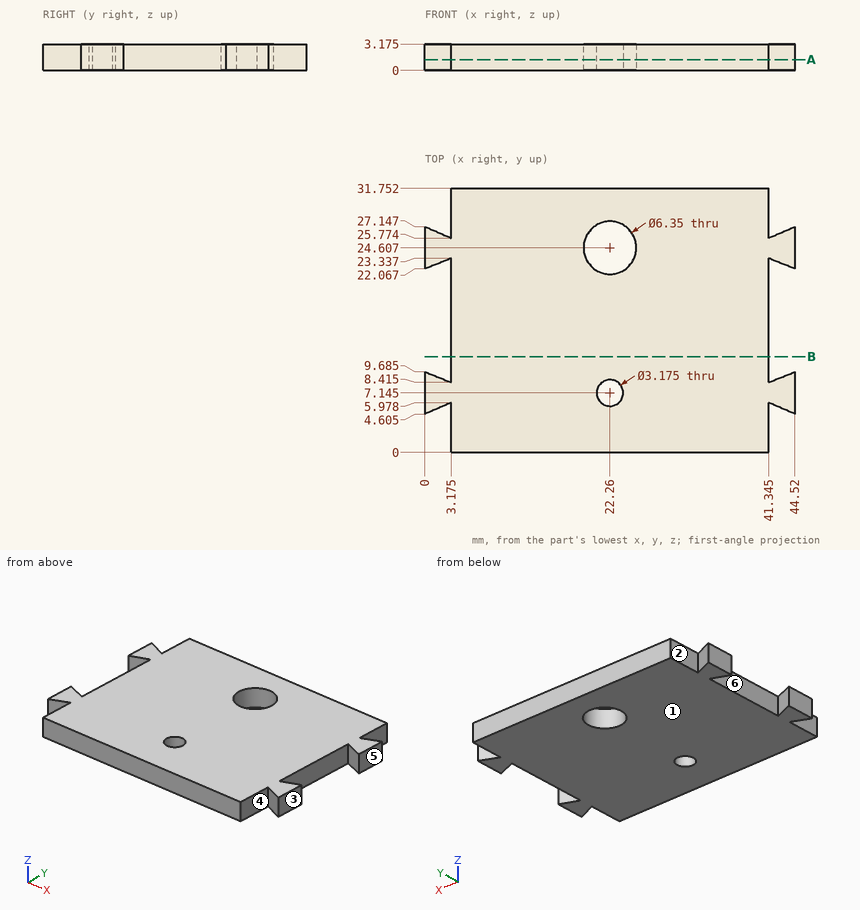
Design review of the part shown in the three views and the two pictorial views. Dimensions are in mm from the part's minimum x, y and z. A direction names the side the tool comes from. Round coordinates to 2 decimals unless told otherwise and drop trailing zeros. Order: outer loops, then holes, each group sorted by start corner. A loop starts at its lowest first (then second) coordinate and runs counter-clockwise, first axis right, second up. Notation, with made-up numbers: (37.25, 32.25) - (67.25, 32.25) arc R11 cw to (67.25, 40.25) - close; hole circle Ø3 at (61, 8). An arc over 180 degrees is marked (long way). Answer in a Markdown table with one row per item.
(1) Machinability: for the marked faces 5 and 6, which of the approach directions +Z, -Z, +X, -X, +Y, -Y give a long, thin tool a straight path to every point of the face, cutting with its end or side? Answer none if there is none.
Result set:
| item | result |
|---|---|
| face 5 | +Z, -Z, +X, +Y, -Y |
| face 6 | +Z, -Z |
(2) Take a section at B-B on y = 11.5. Write out the cut boundary in (x, z) (1 decimal), plus the area to 3 significant figures.
Result set:
| item | result |
|---|---|
| outline | (3.2, 0) - (41.3, 0) - (41.3, 3.2) - (3.2, 3.2) - close |
| area | 121 mm2 |
(3) For line 1 (Y direction, x = 22.5, z = 0.55) (1 decimal); line 2 (X direction, y = 1.5, z = 0.65) (1 decimal); line 3 (X direction, y = 25, z = 2.55), list the stretches that pass through material, from the lowest coordinate up. Write a range as from..to.
Result set:
| item | result |
|---|---|
| line 1 | y = 0..5.6, 8.7..21.4, 27.8..31.8 |
| line 2 | x = 3.2..41.3 |
| line 3 | x = 0..19.11, 25.41..44.52 |
(4) Clearance check with flat-ended pins moving along their axes: P1, Ø1, axis at y = 29, z = 1.5, coming from the +X side (1 decimal); P2, Ø1, axis at y = 13, z = 2, coming from the -X side (3 decimals). State where each tip first meets the part, or that it passes through.
Result set:
| item | result |
|---|---|
| P1 | stops at x = 41.3 |
| P2 | stops at x = 3.175 |
(5) Mouldability with a two-part tool opening along X and no side actions: class the marked faces 1, 2, 3 and 4 as released by +X, released by -X, zero draft, split by the parting line, or undercut.
Result set:
| item | result |
|---|---|
| face 1 | zero draft |
| face 2 | undercut |
| face 3 | released by +X |
| face 4 | undercut |
(6) Take a section at A-A on z = 1.3. Count the separate pieces of the cut face and the enclosed holes in it, plus the area to 3 significant figures.
Result set:
| item | result |
|---|---|
| separate pieces | 1 |
| enclosed holes | 2 |
| area | 1,220 mm2 |
